Read the model definition and answer for the solid it produces. Units are mm, in the model's axes. Face numbers are marked on the shaded views. A direction names the side the tool comes from. Coordinates: 2 decimals unless noted, no trailing zeros. Loops run counter-clockwise (first coordinate to the right, second up) from the corner with the lowest first, then second, coordinate; pieces in that order, holes last. Notation, with made-up numbers: (-9, -19.75) -> (49, -19.75) arc R23 cw to (49, 15.25) -> close; hole circle Ø1 at (-34, 65). An arc over 180 degrees is marked (long way). Answer as a JSON object with one key per item and string values. Group by question number.
1) Consider probe 1 along Y at (x, z) = (-11, 1.4); probe 2 along Y at (x, z) = (10.25, 1.5); probe 3 along X at (y, z) = (11.5, 1.5). Determine where each line is inside the solid, lowest interval first. Write a range as [from, to].
2) Section A-A, the plane y = 11 is taken. Give the vertices of the cut face in (x, z).
3) Determine the mould class of the marked faces 1, 2 and 3 for opening direction X: released by +X, released by -X, zero draft, split by the parting line, or undercut.
4) Flat-ended cylindrical pins translate along their axes: P1, Ø2, axis at x = 6, z = -5, coming from the -Y side; P2, Ø4, axis at x = 11, y = -11, coming from the -Z side; P3, Ø3, axis at x = -3.5, z = -5, coming from the +Y side. Find the tip coordinate at first contact, or state that the pin passes through.
5) Section B-B, the plane x = 0 is taken. Give the vertices of the cut face in (y, z), plus the area to 3 significant figures.
6) Section D-D, the plane z = -5.5 is taken. Give the vertices of the cut face in (x, y).
7) Which of the six approach directions +Z, -Z, +X, -X, +Y, -Y give full straight-line access (tool end or side, diameter ignored) to the marked faces 4 and 5?
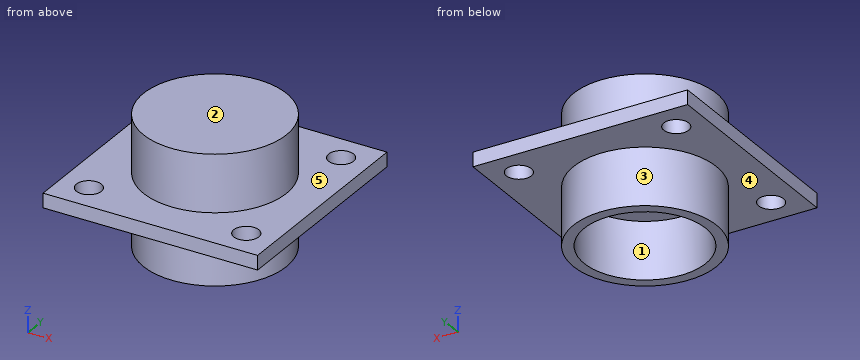
from build123d import *

# Parameters (mm, degrees)
SKETCH_1_W           = 30
SKETCH_1_H           = 30
EXTRUDE_1_DEPTH      = 2
EXTRUDE_2_DEPTH      = 8
EXTRUDE_2_DEPTH_BACK = 10
SKETCH_2_R           = 10
SKETCH_3_R           = 8.5
CUT_EXTRUDE_1_DEPTH  = 8
SKETCH_4_R           = 1.75
CUT_EXTRUDE_2_DEPTH  = 8


with BuildPart() as part:
    # 草图1 → 凸台-拉伸1 (new body)
    with BuildSketch(Plane.XY):
        Rectangle(SKETCH_1_W, SKETCH_1_H)
    extrude(amount=EXTRUDE_1_DEPTH)

    # 草图2 → 凸台-拉伸2 (add, two sides: drawn at the far end of the back side and taken through both)
    with BuildSketch(Plane.XY.offset(2).offset(-EXTRUDE_2_DEPTH_BACK)):
        Circle(SKETCH_2_R)
    extrude(amount=EXTRUDE_2_DEPTH + EXTRUDE_2_DEPTH_BACK)

    # 草图3 → 切除-拉伸1 (cut)
    with BuildSketch(Plane(origin=(0, 0, -8), x_dir=(-1, 0, 0), z_dir=(0, 0, -1))):
        Circle(SKETCH_3_R)
    extrude(amount=-CUT_EXTRUDE_1_DEPTH, mode=Mode.SUBTRACT)

    # 草图4 → 切除-拉伸2 (cut)
    with BuildSketch(Plane(origin=(0, 0, 0), x_dir=(-1, 0, 0), z_dir=(0, 0, -1))):
        with Locations((-11, 11)):
            Circle(SKETCH_4_R)
        with Locations(Location((11, 11, 0), (0, 0, 180))):
            Circle(SKETCH_4_R)
        with Locations((11, -11)):
            Circle(SKETCH_4_R)
        with Locations(Location((-11, -11, 0), (0, 0, 180))):
            Circle(SKETCH_4_R)
    extrude(amount=-CUT_EXTRUDE_2_DEPTH, mode=Mode.SUBTRACT)


solid = part.part
Determined:
{
 "1": {"probe 1": "[-15, -12.75], [-9.25, 9.25], [12.75, 15]", "probe 2": "[-15, -12.58], [-9.42, 9.42], [12.58, 15]", "probe 3": "[-15, -12.68], [-9.32, 9.32], [12.68, 15]"},
 "2": {"outline": "(-15, 0) -> (-12.75, 0) -> (-12.75, 2) -> (-15, 2) -> close; (-9.25, 0) -> (9.25, 0) -> (9.25, 2) -> (-9.25, 2) -> close; (12.75, 0) -> (15, 0) -> (15, 2) -> (12.75, 2) -> close"},
 "3": {"face 1": "undercut", "face 2": "zero draft", "face 3": "split by the parting line"},
 "4": {"P1": "y = -8.66", "P2": "z = 0", "P3": "y = 9.8"},
 "5": {"outline": "(-15, 0) -> (-10, 0) -> (-10, -8) -> (-8.5, -8) -> (-8.5, 0) -> (8.5, 0) -> (8.5, -8) -> (10, -8) -> (10, 0) -> (15, 0) -> (15, 2) -> (10, 2) -> (10, 10) -> (-10, 10) -> (-10, 2) -> (-15, 2) -> close", "area": "244 mm²"},
 "6": {"outline": "circle Ø20 at (0, 0); hole circle Ø17 at (0, 0)"},
 "7": {"face 4": "-Z", "face 5": "+Z"}
}
